Source: three-view drawing plus pictorial views. Frame: mm from the lowest corner of the part. Give positions to 0.01 mm unless a question says otherwise; leave off trailing zeros. Write each loop counter-clockwise with the first axis right and the second up, starting at its lowest first coordinate (ties: lowest second). Pieces come first, ordered by that corner, then holes. Notation, with made-up numbers: (-3.75, -12.75) -> (1.25, -12.75) arc R22 ccw to (1.25, 0.25) -> close; hole circle Ø1 at (-2.5, 41). An arc over 180 degrees is marked (long way). Write item = value, one per line.
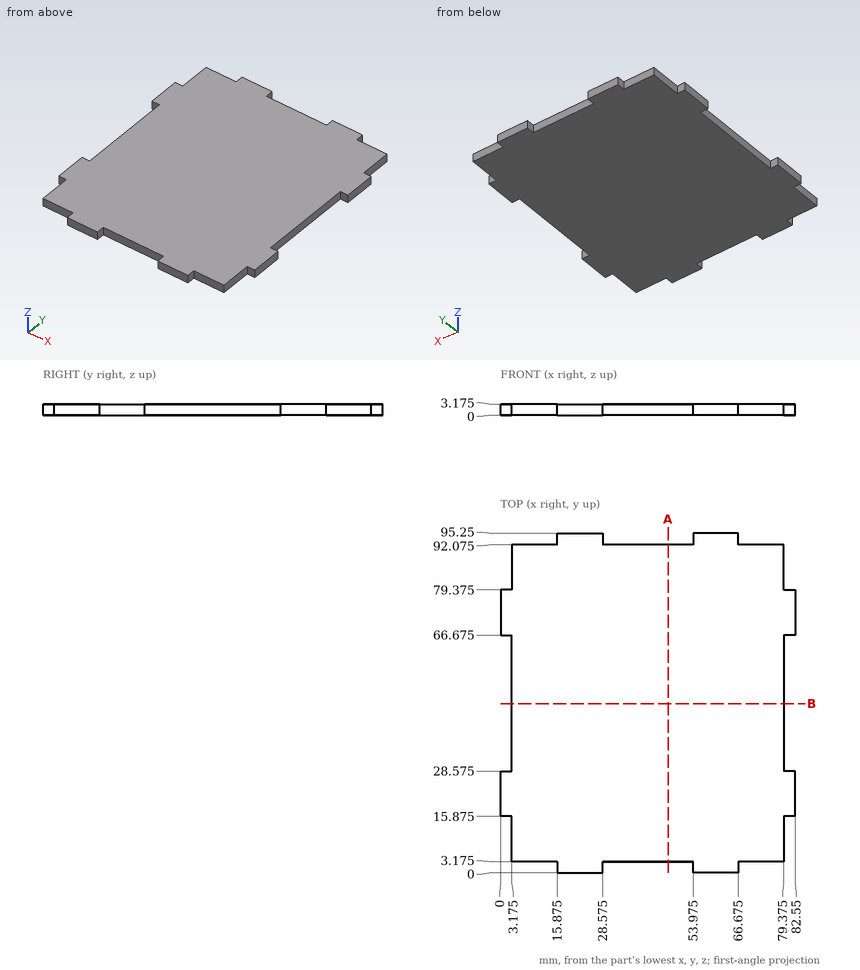
1) Cut plane A-A (x = 47). Return the cut outline in (y, z) (3 decimals), then the cut area to 3 significant figures.
Computed:
outline = (3.175, 0) -> (92.075, 0) -> (92.075, 3.175) -> (3.175, 3.175) -> close
area = 282 mm²
2) Material intervals for L1, parallel to Y at x = 79.5, z = 0.3 (3 decimals); L2, parallel to Y at x = 72, z = 2.65 (3 decimals); L3, parallel to X at y = 38, z = 2.5 (3 decimals), sorted ascending.
Computed:
L1 = 15.875 to 28.575, 66.675 to 79.375
L2 = 3.175 to 92.075
L3 = 3.175 to 79.375
3) Cut plane B-B (y = 47.5). Return the cut outline in (x, z) (3 decimals), then the cut area to 3 significant figures.
Computed:
outline = (3.175, 0) -> (79.375, 0) -> (79.375, 3.175) -> (3.175, 3.175) -> close
area = 242 mm²
4) Contact query for flat-ended pins moving along their axis: pin 1 (1 mm diameter, centred on y = 50, z = 1.5, fed in from -X) (3 decimals); pin 2 (1.6 mm diameter, centred on y = 94, z = 1.5, fed in from -X) (3 decimals); pin 3 (1.6 mm diameter, centred on y = 84.5, z = 2, fed in from +X) (3 decimals). Output: stop coordinate, or through.
Computed:
pin_1 = 3.175
pin_2 = 15.875
pin_3 = 79.375
